from build123d import *

# Parameters (mm, degrees)
CROQUIS1_W              = 13
CROQUIS1_H              = 10.6
SALIENTE_EXTRUIR1_DEPTH = 1.68
CROQUIS2_W              = 2.41
CROQUIS2_H              = 4.48
SALIENTE_EXTRUIR2_DEPTH = 1.3
CROQUIS3_R              = 1.48
CORTAR_EXTRUIR1_DEPTH   = 9.553502207
CROQUIS4_R              = 0.375
CORTAR_EXTRUIR2_DEPTH   = 9.553502207


with BuildPart() as part:
    # Croquis1 → Saliente-Extruir1 (new body)
    with BuildSketch(Plane(origin=(0, 0, 0), x_dir=(1, 0, 0), z_dir=(0, 1, 0))):
        Rectangle(CROQUIS1_W, CROQUIS1_H)
    extrude(amount=SALIENTE_EXTRUIR1_DEPTH)

    # Croquis2 → Saliente-Extruir2 (add)
    with BuildSketch(Plane(origin=(0, 1.68, 0), x_dir=(1, 0, 0), z_dir=(0, 1, 0))):
        with Locations((2.095, -2.31)):
            Rectangle(CROQUIS2_W, CROQUIS2_H)
    extrude(amount=SALIENTE_EXTRUIR2_DEPTH)

    # Croquis3 → Cortar-Extruir1 (cut, through all)
    with BuildSketch(Plane(origin=(0, 1.68, 0), x_dir=(1, 0, 0), z_dir=(0, 1, 0))):
        with Locations(Location((4.12, 2.6, 0), (0, 0, 270))):
            Circle(CROQUIS3_R)
    extrude(amount=-CORTAR_EXTRUIR1_DEPTH, mode=Mode.SUBTRACT)

    # Croquis4 → Cortar-Extruir2 (cut, through all)
    with BuildSketch(Plane(origin=(0, 1.68, 0), x_dir=(1, 0, 0), z_dir=(0, 1, 0))):
        with Locations(Location((-5.5, 3.65, 0), (0, 0, 270))):
            Circle(CROQUIS4_R)
        with Locations(Location((-5.5, 1.11, 0), (0, 0, 270))):
            Circle(CROQUIS4_R)
        with Locations(Location((-5.5, -1.43, 0), (0, 0, 270))):
            Circle(CROQUIS4_R)
        with Locations(Location((-5.5, -3.97, 0), (0, 0, 270))):
            Circle(CROQUIS4_R)
    extrude(amount=-CORTAR_EXTRUIR2_DEPTH, mode=Mode.SUBTRACT)


solid = part.part
Read the model definition and answer for the solid it produces. Units are mm, in the model's axes. A direction names the side the tool comes from. Give positions to 0.01 mm unless a question says otherwise; leave off trailing zeros. Write each loop counter-clockwise with the first axis right and the second up, starting at its lowest first coordinate (ties: lowest second). Pieces come first, ordered by that corner, then holes. Notation, with made-up numbers: M 35.25,-7 L 62.25,-7 A18 ccw 62.25,23 Z; hole C 22.5,44 d2. An arc over 180 degrees is marked long. One line per item, written item: value. Start each with the question number.
(1) Find section C-C (y = 1.05). Determine the outline of the cut face in (x, z) (3 decimals), plus the area to 3 significant figures.
(2) Find section B-B (z = -2.6). Determine the outline of the cut face in (x, y), plus the area to 3 significant figures.
(3) Find the intervals of material crossed by line 1 (X direction, y = 1, z = 3.97) (3 decimals); line 2 (Y direction, x = 0.75, z = -3.75); line 3 (Z direction, x = 4, y = 1.6), in increasing order.
(4) Find section A-A (x = 4.12). Determine the outline of the cut face in (y, z), plus the area to 3 significant figures.
(5) Flat-ended cylindrical pins translate along their axes: pin 1 Ø2.5 at (x, z) = (4.12, -2.6) entering from -Y; pin 2 Ø1.4 at (x, y) = (2.5, 2.5) entering from -Z. Find the tip coordinate at first contact, or state that the pin passes through.
(6) Find section D-D (z = 1.43). Determine the outline of the cut face in (x, y) (3 decimals), plus the area to 3 significant figures.
(7) Determine the mould class of faces 4 (the flat face through (2, 2, 0.07)), 5 (the cylindrical face through (4.6, 0.9, -1.2)), 6 (the flat face through (3.3, 2, 2)), 7 (the flat face through (0, 1, 5.3)) for opening direction Z: pulls with the +Z half, pulls with the -Z half, needs draft (parallel to the pull), parting line crosses it, or undercut.
(8) A tool of negligible diameter and unlimited length cuts with its end or side. For faces 1 (the flat face through (0, 0, 0)), 2 (the flat face through (2, 2, 4.55)), 3 (the flat face through (0.89, 2, 2)), from which of +Z, -Z, +X, -X, +Y, -Y can it reach the whole face along a straight path? Write none if from no direction.
Results below:
1. outline: M -6.5,-5.3 L 6.5,-5.3 L 6.5,5.3 L -6.5,5.3 Z; hole C -5.5,-3.65 d0.75; hole C -5.5,-1.11 d0.75; hole C -5.5,1.43 d0.75; hole C -5.5,3.97 d0.75; hole C 4.12,-2.6 d2.96
1. area: 129 mm^2
2. outline: M -6.5,0 L 2.64,0 L 2.64,1.68 L -6.5,1.68 Z; M 5.6,0 L 6.5,0 L 6.5,1.68 L 5.6,1.68 Z
2. area: 16.9 mm^2
3. line 1: x = -6.5 to -5.875, -5.125 to 6.5
3. line 2: y = 0 to 1.68
3. line 3: z = -5.3 to -4.08, -1.12 to 5.3
4. outline: M 0,-5.3 L 1.68,-5.3 L 1.68,-4.08 L 0,-4.08 Z; M 0,-1.12 L 1.68,-1.12 L 1.68,5.3 L 0,5.3 Z
4. area: 12.8 mm^2
5. pin 1: passes through
5. pin 2: stops at z = 0.07
6. outline: M -6.5,0 L -5.875,0 L -5.875,1.68 L -6.5,1.68 Z; M -5.125,0 L 6.5,0 L 6.5,1.68 L 3.3,1.68 L 3.3,2.98 L 0.89,2.98 L 0.89,1.68 L -5.125,1.68 Z
6. area: 23.7 mm^2
7. face 4: pulls with the -Z half
7. face 5: undercut
7. face 6: needs draft
7. face 7: pulls with the +Z half
8. face 1: +Z, -Z, +X, -X, -Y
8. face 2: +Z, +X, -X, +Y
8. face 3: +Z, -Z, -X, +Y
